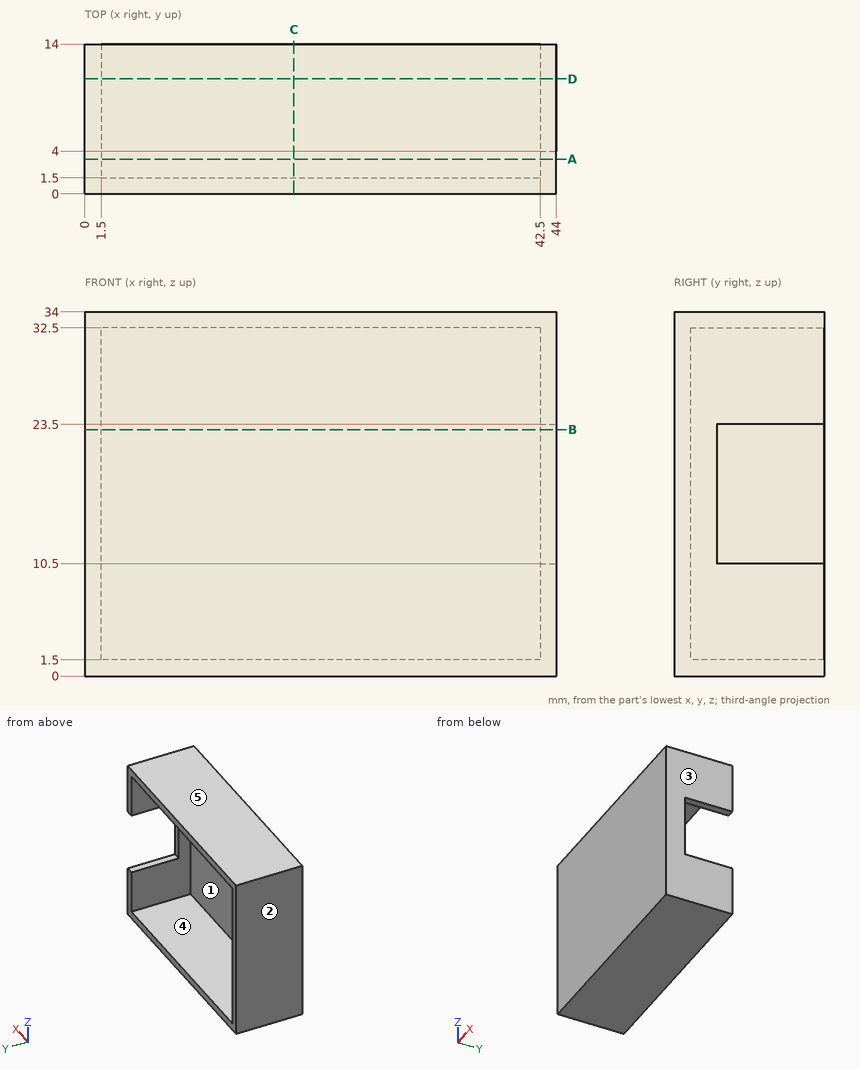
The figure shows three views and two pictorial views of one solid part (mm, origin at its lowest corner). Answer the questions. A direction names the side the tool comes from. Round coordinates to 2 decimals unless told otherwise and drop trailing zeros. Write each loop counter-clockwise with the first axis right and the second up, starting at its lowest first coordinate (ties: lowest second). Pieces come first, ordered by that corner, then holes. Notation, with made-up numbers: M -6.5,0 L 1.5,0 A22 cw 1.5,39 Z; hole C 75.25,89 d5. An arc over 180 degrees is marked long. Use a Markdown table: item, result.
1) For a pull along Z with two mould halves and no side action, classify the marked faces 3, 4 and 5 as pulls with the +Z half, pulls with the -Z half, needs draft (parallel to the pull), parting line crosses it, or undercut.
Answers follow:
| item | result |
|---|---|
| face 3 | needs draft |
| face 4 | undercut |
| face 5 | pulls with the +Z half |
2) The part is cut by section C-C (x = 19.5). Write down the section's boundary in (y, z), plus the area to 3 significant figures.
Answers follow:
| item | result |
|---|---|
| outline | M 0,0 L 14,0 L 14,1.5 L 1.5,1.5 L 1.5,32.5 L 14,32.5 L 14,34 L 0,34 Z |
| area | 88.5 mm2 |
3) A tool of negligible diameter and unlimited length cuts with its end or side. For the marked faces 1 and 2, from which of +Z, -Z, +X, -X, +Y, -Y can it reach the whole face along a straight path? Write none if from no direction.
Answers follow:
| item | result |
|---|---|
| face 1 | +Y |
| face 2 | +Z, -Z, -X, +Y, -Y |
4) The part is cut by section B-B (z = 23). Write down the section's boundary in (x, y), plus the area to 3 significant figures.
Answers follow:
| item | result |
|---|---|
| outline | M 0,0 L 44,0 L 44,4 L 42.5,4 L 42.5,1.5 L 1.5,1.5 L 1.5,14 L 0,14 Z |
| area | 88.5 mm2 |
5) The part is cut by section D-D (y = 10.75). Write down the section's boundary in (x, z).
Answers follow:
| item | result |
|---|---|
| outline | M 0,0 L 44,0 L 44,10.5 L 42.5,10.5 L 42.5,1.5 L 1.5,1.5 L 1.5,32.5 L 42.5,32.5 L 42.5,23.5 L 44,23.5 L 44,34 L 0,34 Z |
6) Straight lines are drawn through the part: line 1 along Z through (x, y) = (15, 4); line 2 along X through (y, z) = (1.75, 10); line 3 along Y through (x, z) = (16.5, 13). For each, find the intervals that lie inside material, in ascending order. Write a range as [from, to].
Answers follow:
| item | result |
|---|---|
| line 1 | z = [0, 1.5], [32.5, 34] |
| line 2 | x = [0, 1.5], [42.5, 44] |
| line 3 | y = [0, 1.5] |
7) Flat-ended cylindrical pins translate along their axes: pin 1 (15.5 mm diameter, centred on x = 28.5, z = 18.5, fed in from +Y); pin 2 (1.6 mm diameter, centred on x = 43, z = 19, fed in from +Y). Find the tip coordinate at first contact, or state that the pin passes through.
Answers follow:
| item | result |
|---|---|
| pin 1 | stops at y = 1.5 |
| pin 2 | stops at y = 4 |
8) The part is cut by section A-A (y = 3.25). Write down the section's boundary in (x, z).
Answers follow:
| item | result |
|---|---|
| outline | M 0,0 L 44,0 L 44,34 L 0,34 Z; hole M 1.5,1.5 L 42.5,1.5 L 42.5,32.5 L 1.5,32.5 Z |
